Part print with two shaded views. Sizes in mm from the minimum x, y, z corner. A direction names the side the tool comes from. Round coordinates to 2 decimals unless told otherwise and drop trailing zeros. Write each loop counter-clockwise with the first axis right and the second up, starting at its lowest first coordinate (ties: lowest second). Pieces come first, ordered by that corner, then holes.
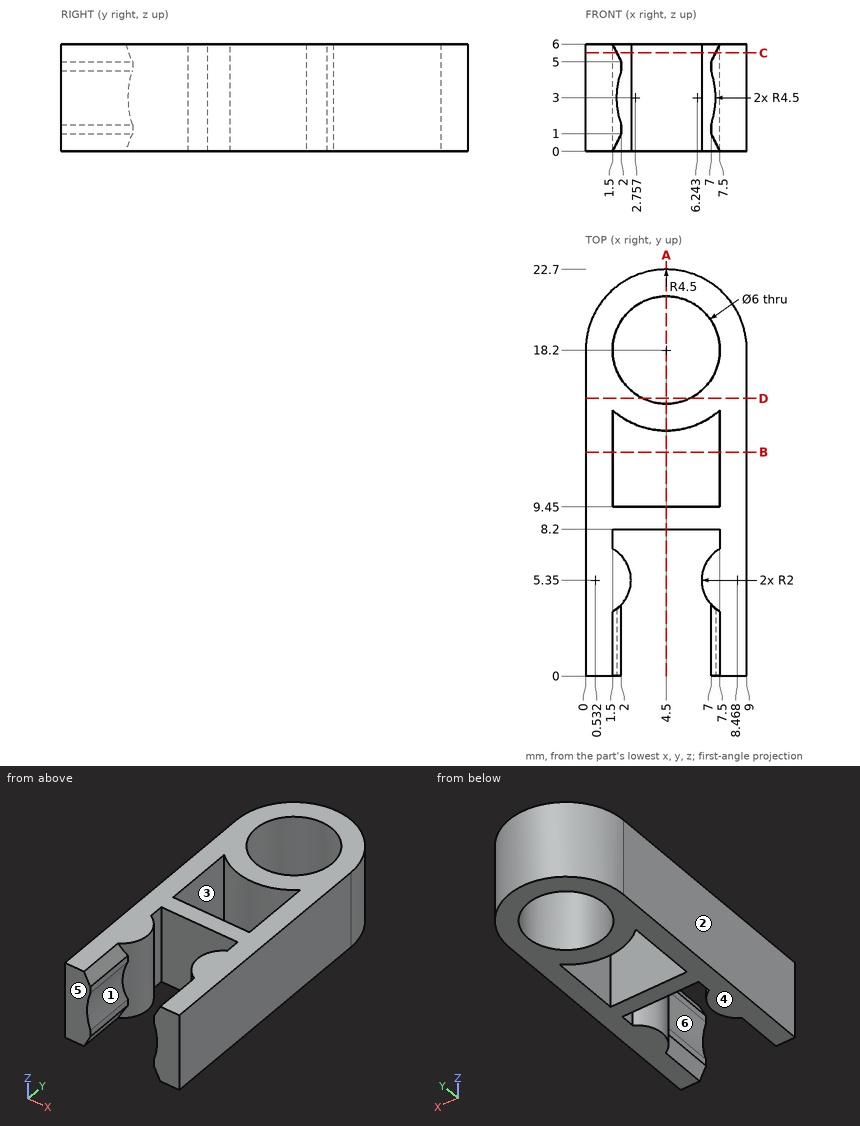
Q1. Which spindle directions (+Z, -Z, +X, -X, +Y, -Y) get a long thin tool onto all of the face, cutting with end or side? Do the marked faces 1, 2 and 3. Say none if no direction does.
Values follow:
face 1: -Y
face 2: +Z, -Z, -X, +Y, -Y
face 3: +Z, -Z
Q2. Cut at C-C on z = 5.5. Write the cut outline in (x, y).
Values follow:
outline: (0, 0) - (1.75, 0) - (1.75, 3.76) arc R2 ccw to (1.5, 7.1) - (1.5, 8.2) - (7.5, 8.2) - (7.5, 7.1) arc R2 ccw to (7.25, 3.76) - (7.25, 0) - (9, 0) - (9, 18.2) arc R4.5 ccw to (0, 18.2) - close; hole (1.5, 9.45) - (7.5, 9.45) - (7.5, 14.85) arc R4.5 cw to (1.5, 14.85) - close; hole circle Ø6 at (4.5, 18.2)
Q3. Drop flat-ended pins along their axis: pin 1 (3 mm diameter, centred on x = 5.5, z = 2.5, fed in from +Y); pin 2 (2 mm diameter, centred on x = 7.5, z = 2, fed in from +Y); pin 3 (1.8 mm diameter, centred on x = 3.5, z = 2, fed in from -Y); pin 4 (3.5 mm diameter, centred on x = 4.5, y = 18.2, fed in from +Z). Give the stop position or say it passes through.
Values follow:
pin 1: stops at y = 22.7
pin 2: stops at y = 22.23
pin 3: stops at y = 8.2
pin 4: passes through
Q4. Cut at D-D on y = 15.5. Write the cut outline in (x, z).
Values follow:
outline: (0, 0) - (3.19, 0) - (3.19, 6) - (0, 6) - close; (5.81, 0) - (9, 0) - (9, 6) - (5.81, 6) - close
Q5. Cut at B-B on y = 12.5. Write the cut outline in (x, z), plus the area to 3 significant figures.
Values follow:
outline: (0, 0) - (1.5, 0) - (1.5, 6) - (0, 6) - close; (7.5, 0) - (9, 0) - (9, 6) - (7.5, 6) - close
area: 18.0 mm2
Q6. Cut at A-A on x = 4.5. Write the cut outline in (y, z).
Values follow:
outline: (8.2, 0) - (9.45, 0) - (9.45, 6) - (8.2, 6) - close; (13.7, 0) - (15.2, 0) - (15.2, 6) - (13.7, 6) - close; (21.2, 0) - (22.7, 0) - (22.7, 6) - (21.2, 6) - close
Q7. Wall check: L1, parallel to Y at x = 4.5, z = 4.6; L2, parallel to X at y = 12, z = 0.5; L3, parallel to X at y = 2, z = 1.25. Give the ranges that are in metal, low to high.
Values follow:
L1: y = 8.2 to 9.45, 13.7 to 15.2, 21.2 to 22.7
L2: x = 0 to 1.5, 7.5 to 9
L3: x = 0 to 2, 7 to 9
Q8. Mould opens along Z. For the marked faces 4, 5 and 6 say: +Z half, -Z half, draft (parallel to the pull), parting line (faces both ways), or undercut.
Values follow:
face 4: -Z half
face 5: draft
face 6: undercut
